For this review, take the finished solid that the model builds, in its own axes (mm). Face numbers are marked on the shaded views. A direction names the side the tool comes from. Round coordinates to 2 decimals unless told otherwise and drop trailing zeros. Write each loop counter-clockwise with the first axis right and the second up, starting at its lowest first coordinate (ties: lowest second). Pieces come first, ordered by that corner, then holes. Notation, with made-up numbers: M 15.25,20 L 59.25,20 A31 ccw 59.25,49 Z; hole C -18,78.5 d3. An arc over 180 degrees is marked long. Write each question's results on one line, items separated by ' | '. Start each with the question number.
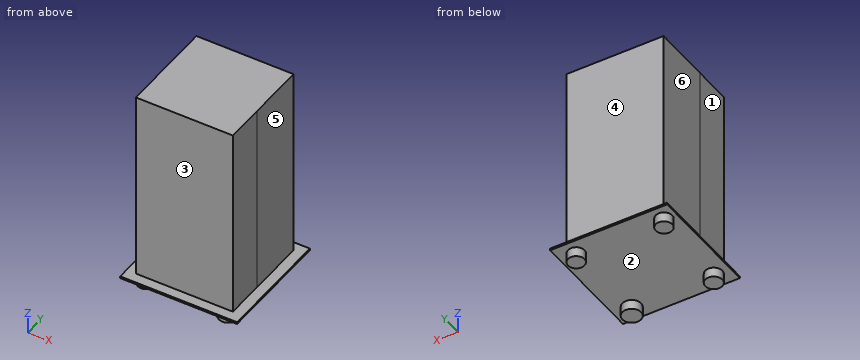
```python
from build123d import *

# Parameters (mm, degrees)
F1_W      = 63.300895
F1_H      = 127
F2_DEPTH  = 25.4
F2_FACE_W = 63.300894
F2_FACE_H = 127
F3_DEPTH  = 38.1
F0_W      = 76.2
F0_H      = 76.2
F0_W_2    = 63.5
F0_H_2    = 63.5
F4_DEPTH  = 1.27
F5_R      = 5.570657
F5_R_2    = 6.11713
F5_R_3    = 5.40011
F5_R_4    = 5.400115
F6_DEPTH  = 6.35


with BuildPart() as f2:
    # F1 (on Front) → F2 (new body)
    with BuildSketch(Plane.XZ):
        with Locations((0.75961, 63.5)):
            Rectangle(F1_W, F1_H)
    extrude(amount=F2_DEPTH)

    # F2_face (on face) → F3 (join)
    with BuildSketch(Plane(origin=(0.75961, 0, 63.5), x_dir=(1, 0, 0), z_dir=(0, 1, 0))):
        Rectangle(F2_FACE_W, F2_FACE_H)
    extrude(amount=F3_DEPTH)

    # F0 (on Top) → F4 (join)
    with BuildSketch(Plane.XY):
        with Locations((1.143001, 6.07413)):
            Rectangle(F0_W, F0_H)
        with Locations((1.143001, 6.07413)):
            Rectangle(F0_W_2, F0_H_2, mode=Mode.SUBTRACT)
        with Locations((1.143001, 6.07413)):
            Rectangle(F0_W_2, F0_H_2)
    extrude(amount=F4_DEPTH)

    # F5 (on face) → F6 (join)
    with BuildSketch(Plane(origin=(0, 0, 0), x_dir=(1, 0, 0), z_dir=(0, 0, -1))):
        with Locations((-26.67, 21.333355)):
            Circle(F5_R)
        with Locations((27.178001, 21.841355)):
            Circle(F5_R_2)
        with Locations((28.448002, -34.292646)):
            Circle(F5_R_3)
        with Locations((-28.956, -34.546643)):
            Circle(F5_R_4)
    extrude(amount=F6_DEPTH)


solid = f2.part
```
Item 1: We need section D-D on x = -26.67. State the section outline as (y, z) points, then the cut area to 3 significant figures.
Item 2: For probe 1 along X at (y, z) = (7, 106); probe 2 along Y at (x, z) = (-0.5, 67.5); probe 3 along Z at (x, y) = (-8.5, 40), list the stretches that pass through material, from the lowest coordinate up.
Item 3: We need section C-C on y = -14. State the section outline as (x, z) points, then the cut area to 3 significant figures.
Item 4: We need section A-A on x = 3. State the section outline as (y, z) points.
Item 5: Insertion check: P1, Ø20.5, axis at y = -8.5, z = 41, coming from the +X side; P2, Ø19, axis at y = 19.5, z = 80, coming from the -X side; P3, Ø4, axis at x = -24.5, z = 107.5, coming from the +Y side. Each pin has a flat end and moves straight along its axis. Give the tip position at first contact, or say it passes through.
Item 6: We need section B-B on z = 116. State the section outline as (x, y) points, then the cut area to 3 significant figures.
Item 7: For the marked faces 4, 5 and 6, list the 3-axis set-ups (+Z, -Z, +X, -X, +Y, -Y) from which the entire face can be reached by the end or side of a thin tool; tool diameter is ignored.
Item 8: Mouldability with a two-part tool opening along X and no side actions: class the marked faces 1, 2 and 3 as pulls with the +X half, pulls with the -X half, needs draft (parallel to the pull), parting line crosses it, or undercut.
Numbers:
1) outline: M -32.03,0 L -26.9,0 L -26.9,-6.35 L -15.76,-6.35 L -15.76,0 L 29.65,0 L 29.65,-6.35 L 39.44,-6.35 L 39.44,0 L 44.17,0 L 44.17,1.27 L 38.1,1.27 L 38.1,127 L -25.4,127 L -25.4,1.27 L -32.03,1.27 Z | area: 8,210 mm^2
2) probe 1: x = -30.89 to 32.41 | probe 2: y = -25.4 to 38.1 | probe 3: z = 0 to 1.27
3) outline: M -36.96,0 L 39.24,0 L 39.24,1.27 L 32.41,1.27 L 32.41,127 L -30.89,127 L -30.89,1.27 L -36.96,1.27 Z | area: 8,060 mm^2
4) outline: M -32.03,0 L 44.17,0 L 44.17,1.27 L 38.1,1.27 L 38.1,127 L -25.4,127 L -25.4,1.27 L -32.03,1.27 Z
5) P1: stops at x = 32.41 | P2: stops at x = -30.89 | P3: stops at y = 38.1
6) outline: M -30.89,-25.4 L 32.41,-25.4 L 32.41,38.1 L -30.89,38.1 Z | area: 4,020 mm^2
7) face 4: +Z, +X, -X, +Y | face 5: +Z, +X, +Y, -Y | face 6: +Z, -X, +Y, -Y
8) face 1: pulls with the -X half | face 2: undercut | face 3: needs draft
